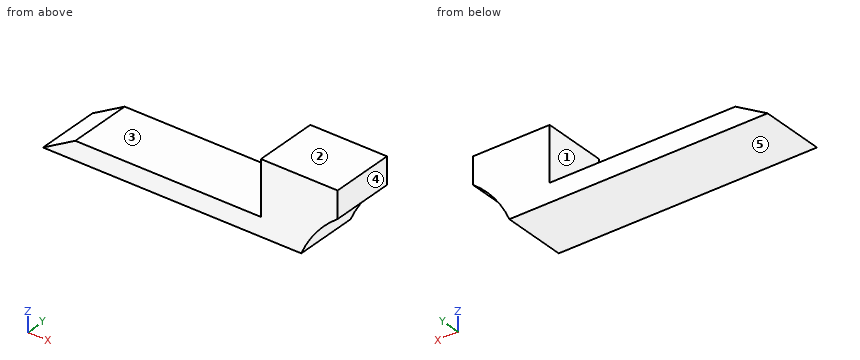
from build123d import *

# Parameters (mm, degrees)
F1_DEPTH = 7.95


with BuildPart() as f1:
    # F0 (on Front) → F1 (new body)
    with BuildSketch(Plane.XZ):
        with BuildLine():
            Line((4, 2.309401), (0, 0))
            Line((0, 0), (25.413539, 0))
            Line((25.413539, 0), (32, 0))
            ThreePointArc((32, 0), (33.863776, 3.157224), (36.5, 5.705172))
            Line((36.5, 5.705172), (36.5, 9.02))
            Line((36.5, 9.02), (27, 9.02))
            Line((27, 9.02), (27, 4.098076))
            Line((27, 4.098076), (27, 2.309401))
            Line((27, 2.309401), (4, 2.309401))
        make_face()
    extrude(amount=F1_DEPTH)


solid = f1.part
Verification items for the finished model (mm, model axes). Face numbers are marked on the shaded views. A direction names the side the tool comes from. Coordinates: 2 decimals unless noted, no trailing zeros. Order: outer loops, then holes, each group sorted by start corner. A loop starts at its lowest first (then second) coordinate and runs counter-clockwise, first axis right, second up. Notation, with made-up numbers: (66, 58) -> (93, 58) arc R15 cw to (93, 85) -> close; hole circle Ø6 at (76.5, 35). An arc over 180 degrees is marked (long way). Use CSV: the item, a comma, the result in double quotes. Start each with the question number.
Q1. Draft check along Z on the marked faces 3, 4 and 5. Enter one of: +Z half, -Z half, draft (parallel to the pull), parting line (faces both ways), or undercut.
Q2. Section check A-A, the plane y = -2.5. Record the cut outline in (x, z), and give its area (3 significant figures).
Q3. Depth check by flat-ended pin: P1, Ø2, axis at y = -2.5, z = 4.5, coming from the -X side. Enter the tip coordinate at first touch or a pass-through.
Q4. Section check C-C, the plane z = 6.25. Record the cut outline in (x, y), and give its area (3 significant figures).
Q5. Tool access check on the marked faces 1 and 2. Record the directions out of +Z, -Z, +X, -X, +Y, -Y that give a thin tool (end or side, any length) a straight path to the whole face; none if there is none.
Q6. Section check B-B, the plane x = 17. Record the cut outline in (y, z), and give its area (3 significant figures).
Q7. Thickness scan on line 1 along Z through (x, y) = (21, -3.25); line 2 along X through (y, z) = (-6, 7.75); line 3 along Z through (x, y) = (33, -3). Record the ranges inside material, lowest first.
Returned:
1,face 3,"+Z half"
1,face 4,"draft"
1,face 5,"-Z half"
2,outline,"(0, 0) -> (32, 0) arc R13.66 cw to (36.5, 5.71) -> (36.5, 9.02) -> (27, 9.02) -> (27, 2.31) -> (4, 2.31) -> close"
2,area,"128 mm^2"
3,P1,"stops at x = 27"
4,outline,"(27, -7.95) -> (36.5, -7.95) -> (36.5, 0) -> (27, 0) -> close"
4,area,"75.5 mm^2"
5,face 1,"+Z, -X, +Y, -Y"
5,face 2,"+Z, +X, -X, +Y, -Y"
6,outline,"(-7.95, 0) -> (0, 0) -> (0, 2.31) -> (-7.95, 2.31) -> close"
6,area,"18.4 mm^2"
7,line 1,"z = 0 to 2.31"
7,line 2,"x = 27 to 36.5"
7,line 3,"z = 1.93 to 9.02"
